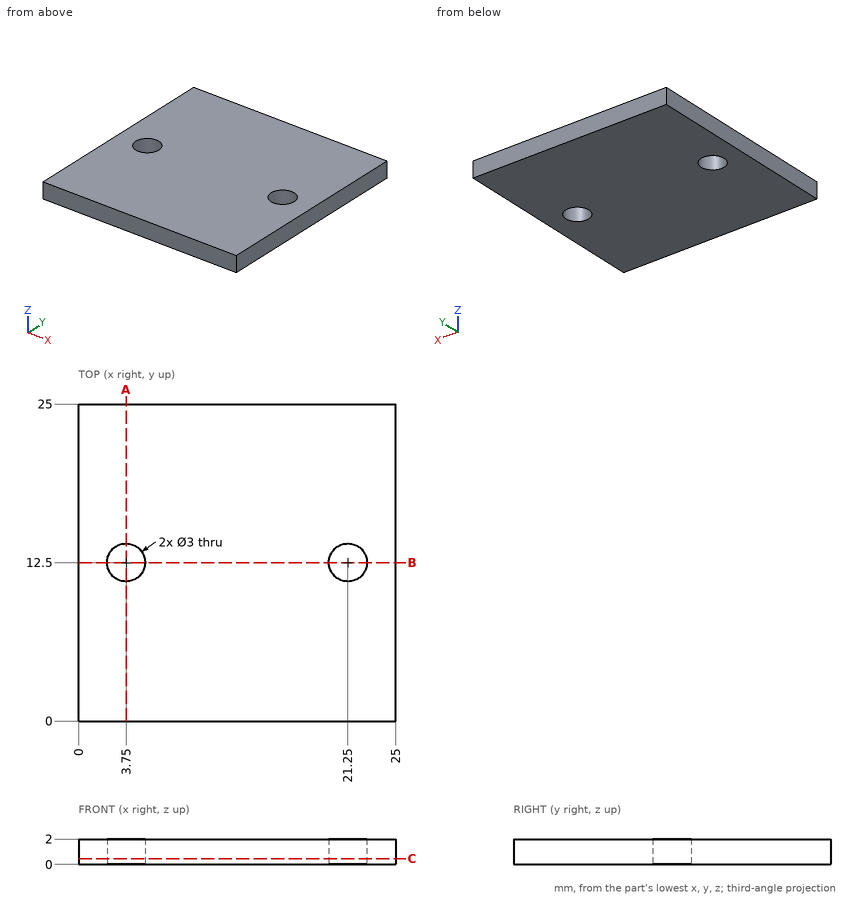
Answer from the drawing. Dimensions are ordinates in mm from the lowest x, y and z of the part. Coordinates: 2 decimals unless noted, no trailing zeros. Loops run counter-clockwise (first coordinate to the right, second up) from the corner with the lowest first, then second, coordinate; pieces in that order, holes last.
Q1. Each of these flat-tipped pins is pushed along its axis until it touches: pin 1 Ø12 at (x, y) = (21, 15.5) entering from -Z; pin 2 Ø2.5 at (x, y) = (21.25, 12.5) entering from +Z. Where does it stop, or does it pass through?
Q2. The part is cut by section B-B on y = 12.5. Write down the section's boundary in (x, z), and give its area (3 significant figures).
Q3. Consider probe 1 along Y at (x, z) = (3.75, 0.9); probe 2 along Y at (x, z) = (20.75, 0.5). Determine where each line is inside the solid, lowest interval first.
Q4. The part is cut by section A-A on x = 3.75. Write down the section's boundary in (y, z).
Q5. The part is cut by section C-C on z = 0.45. Write down the section's boundary in (x, y).
Results below:
1. pin 1: stops at z = 0
1. pin 2: passes through
2. outline: (0, 0) - (2.25, 0) - (2.25, 2) - (0, 2) - close; (5.25, 0) - (19.75, 0) - (19.75, 2) - (5.25, 2) - close; (22.75, 0) - (25, 0) - (25, 2) - (22.75, 2) - close
2. area: 38.0 mm2
3. probe 1: y = 0 to 11, 14 to 25
3. probe 2: y = 0 to 11.09, 13.91 to 25
4. outline: (0, 0) - (11, 0) - (11, 2) - (0, 2) - close; (14, 0) - (25, 0) - (25, 2) - (14, 2) - close
5. outline: (0, 0) - (25, 0) - (25, 25) - (0, 25) - close; hole circle Ø3 at (3.75, 12.5); hole circle Ø3 at (21.25, 12.5)
